from build123d import *

# Parameters (mm, degrees)
SKETCH1_R                = 2.5
BOSS_EXTRUDE1_DEPTH      = 4
BOSS_EXTRUDE3_DEPTH      = 2.5
BOSS_EXTRUDE4_DEPTH      = 3.5
BOSS_EXTRUDE4_DEPTH_BACK = 4
SKETCH5_R                = 5


with BuildPart() as part:
    # Sketch1 → Boss-Extrude1 (new body)
    with BuildSketch(Plane.XY):
        Circle(SKETCH1_R)
    extrude(amount=BOSS_EXTRUDE1_DEPTH)

    # Sketch3 → Boss-Extrude3 (add)
    with BuildSketch(Plane.XY.offset(4)):
        with BuildLine():
            Line((0, 10), (300, 10))
            ThreePointArc((300, 10), (310, 0), (300, -10))
            Line((300, -10), (0, -10))
            ThreePointArc((0, -10), (-10, 0), (0, 10))
        make_face()
        with BuildLine():
            Line((15, 3), (110, 3))
            ThreePointArc((110, 3), (113, 0), (110, -3))
            Line((110, -3), (15, -3))
            ThreePointArc((15, -3), (12, 0), (15, 3))
        make_face(mode=Mode.SUBTRACT)
        with BuildLine():
            Line((285, 3), (190, 3))
            ThreePointArc((190, 3), (187, 0), (190, -3))
            Line((190, -3), (285, -3))
            ThreePointArc((285, -3), (288, 0), (285, 3))
        make_face(mode=Mode.SUBTRACT)
    extrude(amount=BOSS_EXTRUDE3_DEPTH)

    # Sketch5 → Boss-Extrude4 (add, two sides: drawn at the far end of the back side and taken through both)
    with BuildSketch(Plane(origin=(0, 0, 4), x_dir=(-1, 0, 0), z_dir=(0, 0, -1)).offset(-BOSS_EXTRUDE4_DEPTH_BACK)):
        with Locations((-300, 0)):
            Circle(SKETCH5_R)
    extrude(amount=BOSS_EXTRUDE4_DEPTH + BOSS_EXTRUDE4_DEPTH_BACK)


solid = part.part
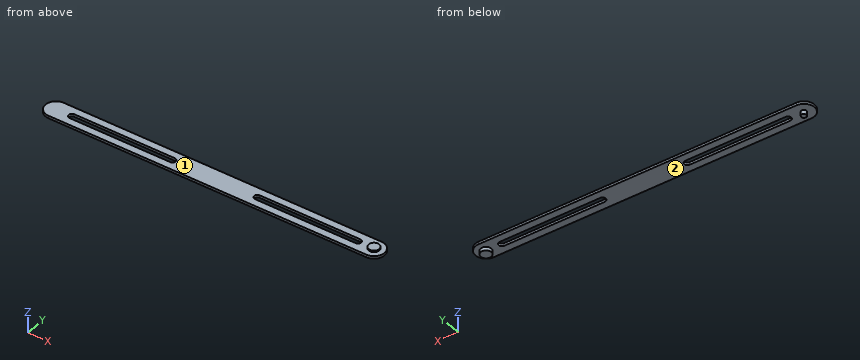
Can you work these out from the model? Positions are in its coordinate system, mm. Face numbers are marked on the shaded views. Coordinates: 2 decimals unless noted, no trailing zeros. Write each loop counter-clockwise with the first axis right and the second up, starting at its lowest first coordinate (ties: lowest second). Pieces come first, ordered by that corner, then holes. Notation, with made-up numbers: M -3.75,8 L 13.25,8 A13 cw 13.25,32 Z; hole C 24.5,47 d11. An arc over 180 degrees is marked long. Use one line per item in the form item = value.
Q1. We'd pull the mould along Z, two halves only. Please class the marked faces 1 and 2: +Z half, -Z half, draft (parallel to the pull), parting line (faces both ways), or undercut.
Model answer:
face_1 = +Z half
face_2 = -Z half
Q2. If we section it at A-A (x = 44.5): Write out the boundary of the cut face in (y, z).
Model answer:
outline = M -10,4 L -3,4 L -3,6.5 L -10,6.5 Z; M 3,4 L 10,4 L 10,6.5 L 3,6.5 Z
Q3. I need wall thicknesses on line 1 along X through (y, z) = (-2.5, 5.5); line 2 along Y through (x, z) = (90, 6.25); line 3 along Z through (x, y) = (261, 6.25). Which ranges of each line are inside material? Lowest first, please. Write a range as from..to.
Model answer:
line_1 = -9.68..13.34, 111.66..188.34, 286.66..309.68
line_2 = -10..-3, 3..10
line_3 = 4..6.5
Q4. If we section it at C-C (x = 165.5): Write out the boundary of the cut face in (y, z).
Model answer:
outline = M -10,4 L 10,4 L 10,6.5 L -10,6.5 Z
Q5. For P1, Ø12, axis at x = 126.5, y = -8, coming from the +Z side; P2, Ø2, axis at x = 174, y = -5.5, coming from the -Z side; P3, Ø11, axis at x = 301.5, y = 0.5, coming from the -Z side, each with a flat end and sliding along its axis, tell me the tip position at first contact or that it passes through.
Model answer:
P1 = 6.5
P2 = 4
P3 = 0.5
Q6. If we section it at B-B (z = 2): Write out the boundary of the cut face in (x, y), then the cut area to 3 significant figures.
Model answer:
outline = C 0,0 d5; C 300,0 d10
area = 98.2 mm^2
